For this review, take the finished solid that the model builds, in its own axes (mm). A direction names the side the tool comes from. Coordinates: 2 decimals unless noted, no trailing zeros. Loops run counter-clockwise (first coordinate to the right, second up) from the corner with the lowest first, then second, coordinate; pieces in that order, holes last. Notation, with made-up numbers: M 50,34 L 107,34 A29 cw 107,56 Z; hole C 56.25,88 d3. An arc over 180 degrees is marked long. Put each result on its own line as item: value.
Autodesk Inventor part; units mm, degrees
ref_plane "YZ Plane" through (0, 0, 0) normal (1, 0, 0) x (0, 1, 0)
ref_plane "XZ Plane" through (0, 0, 0) normal (0, 1, 0) x (-1, 0, 0)
ref_plane "XY Plane" through (0, 0, 0) normal (0, 0, 1) x (1, 0, 0)
sketch "Sketch1" plane through (0, 0, 0) normal (0, 1, 0) x (-1, 0, 0)
  line L0 (0, 0) -> (-60, 0)
  line L1 (-60, 0) -> (-60, -48)
  line L2 (-60, -48) -> (0, -48)
  line L3 (0, -48) -> (0, 0)
  line L4 (-8, -18) -> (-52, -18)
  line L5 (-52, -18) -> (-52, -12)
  line L6 (-52, -12) -> (-8, -12)
  line L7 (-8, -12) -> (-8, -18)
  dimension "d0" = 60
  dimension "d1" = 48
  dimension "d14" = 44
  dimension "d15" = 6
  dimension "d16" = 8
  dimension "d17" = 12
extrude "Extrusion1" add sketch "Sketch1" along normal blind 4
sketch "Sketch2" plane through (0, 4, 0) normal (0, 1, 0) x (1, 0, 0)
  line L0 (0, 0) -> (60, 0) construction
  line L1 (60, 0) -> (60, 48) construction
  line L2 (60, 48) -> (0, 48) construction
  line L3 (0, 48) -> (0, 0) construction
  line L4 (4, 44) -> (56, 44) construction
  line L5 (56, 44) -> (56, 4) construction
  line L6 (56, 4) -> (4, 4) construction
  line L7 (4, 4) -> (4, 44) construction
  line L8 (60, 48) -> (0, 48) construction
  line L9 (30, 48) -> (30, 0) construction
  line L10 (0, 0) -> (60, 0) construction
  line L11 (0, 48) -> (0, 0) construction
  line L12 (0, 24) -> (60, 24) construction
  line L13 (60, 0) -> (60, 48) construction
  line L14 (0, 28) -> (4, 28)
  line L15 (0, 36) -> (4, 36)
  line L16 (10, 48) -> (10, 44)
  line L17 (10, 44) -> (18, 44)
  line L18 (18, 44) -> (18, 48)
  line L19 (18, 48) -> (10, 48)
  line L20 (26, 48) -> (26, 44)
  line L21 (26, 44) -> (30, 44)
  line L22 (26, 48) -> (30, 48)
  line L23 (0, 36) -> (0, 28)
  line L24 (4, 28) -> (4, 36)
  line L25 (60, 28) -> (56, 28)
  line L26 (60, 36) -> (56, 36)
  line L27 (50, 48) -> (50, 44)
  line L28 (50, 44) -> (42, 44)
  line L29 (42, 44) -> (42, 48)
  line L30 (42, 48) -> (50, 48)
  line L31 (34, 48) -> (34, 44)
  line L32 (34, 44) -> (30, 44)
  line L33 (34, 48) -> (30, 48)
  line L34 (60, 36) -> (60, 28)
  line L35 (56, 28) -> (56, 36)
  line L36 (60, 0) -> (0, 0) construction
  line L37 (4, 4) -> (56, 4) construction
  line L38 (60, 0) -> (0, 0) construction
  line L39 (0, 20) -> (4, 20)
  line L40 (0, 12) -> (4, 12)
  line L41 (10, 0) -> (10, 4)
  line L42 (10, 4) -> (18, 4)
  line L43 (18, 4) -> (18, 0)
  line L44 (18, 0) -> (10, 0)
  line L45 (26, 0) -> (26, 4)
  line L46 (26, 4) -> (30, 4)
  line L47 (26, 0) -> (30, 0)
  line L48 (0, 12) -> (0, 20)
  line L49 (4, 20) -> (4, 12)
  line L50 (34, 0) -> (34, 4)
  line L51 (34, 4) -> (30, 4)
  line L52 (34, 0) -> (30, 0)
  line L53 (42, 4) -> (42, 0)
  line L54 (50, 4) -> (42, 4)
  line L55 (42, 0) -> (50, 0)
  line L56 (50, 0) -> (50, 4)
  line L57 (56, 20) -> (56, 12)
  line L58 (60, 12) -> (56, 12)
  line L59 (60, 12) -> (60, 20)
  line L60 (60, 20) -> (56, 20)
  dimension "d4" = 4
  dimension "d7" = 8
  dimension "d8" = 8
  dimension "d9" = 4
  dimension "d10" = 8
  dimension "d11" = 4
extrude "Extrusion2" cut sketch "Sketch2" against normal up to surface (4 mm away)
properties part number "left" material "PBT Plastic Black"
(1) Add section B-B (z = -45). Write out the cut boundary in (x, y).
Determined:
outline: M 0,0 L 10,0 L 10,4 L 0,4 Z; M 18,0 L 26,0 L 26,4 L 18,4 Z; M 34,0 L 42,0 L 42,4 L 34,4 Z; M 50,0 L 60,0 L 60,4 L 50,4 Z
(2) Draft analysis for pull direction Z (two halves, no side actions). For faces 1 (the flat face through (30, 2, -12)), 2 (the flat face through (14, 2, -44)), 3 (the flat face through (60, 2, -24)), 4 (the flat face through (5, 2, 0)), state which applies: +Z half, -Z half, draft (parallel to the pull), parting line (faces both ways), or undercut.
Determined:
face 1: undercut
face 2: -Z half
face 3: draft
face 4: +Z half
(3) Add section C-C (z = -16). Write out the cut boundary in (x, y), plus the area to 3 significant figures.
Determined:
outline: M 4,0 L 8,0 L 8,4 L 4,4 Z; M 52,0 L 56,0 L 56,4 L 52,4 Z
area: 32.0 mm^2
(4) Wall thickness on line 1 along X through (y, z) = (3.7, -3); line 2 along Z through (x, y) = (57, 0.4); line 3 along Z through (x, y) = (14, 2.9): over which ranges is each line inside the solid? List them lowest first. Write a range as [from, to].
Determined:
line 1: x = [0, 10], [18, 26], [34, 42], [50, 60]
line 2: z = [-48, -36], [-28, -20], [-12, 0]
line 3: z = [-44, -18], [-12, -4]
(5) Add section A-A (x = 23.5). Write out the cut boundary in (y, z).
Determined:
outline: M 0,-48 L 4,-48 L 4,-18 L 0,-18 Z; M 0,-12 L 4,-12 L 4,0 L 0,0 Z
(6) Add section D-D (z = -35). Write out the cut boundary in (x, y), plus the area to 3 significant figures.
Determined:
outline: M 4,0 L 56,0 L 56,4 L 4,4 Z
area: 208 mm^2
(7) For pin 1 (1.2 mm diameter, centred on x = 12, y = 3, fed in from +Z); pin 2 (2 mm diameter, centred on y = 2, z = -18, fed in from -X), all flat-tipped, find the tip position at first contact; note any pin that passes through.
Determined:
pin 1: stops at z = -4
pin 2: stops at x = 4
(8) Tool access review of faces 5 (the flat face through (26, 2, -46)), 6 (the flat face through (46, 2, -4)), 7 (the flat face through (58, 2, -20)): name each direction out of +Z, -Z, +X, -X, +Y, -Y from which nothing blocks a thin tool from reaching the whole face with its end or side.
Determined:
face 5: -Z, +Y, -Y
face 6: +Z, +Y, -Y
face 7: +X, +Y, -Y
